```python
from build123d import *

# Parameters (mm, degrees)
F0_R     = 2
F0_R_2   = 12.5
F1_DEPTH = 1


with BuildPart() as f1:
    # F0 (on Top) → F1 (new body)
    with BuildSketch(Plane.XY):
        with BuildLine():
            ThreePointArc((21.15, 16.15), (19.685534, 19.685534), (16.15, 21.15))
            Line((16.15, 21.15), (-16.15, 21.15))
            ThreePointArc((-16.15, 21.15), (-19.685534, 19.685534), (-21.15, 16.15))
            Line((-21.15, 16.15), (-21.15, -16.15))
            ThreePointArc((-21.15, -16.15), (-19.685534, -19.685534), (-16.15, -21.15))
            Line((-16.15, -21.15), (16.15, -21.15))
            ThreePointArc((16.15, -21.15), (19.685534, -19.685534), (21.15, -16.15))
            Line((21.15, -16.15), (21.15, 16.15))
        make_face()
        with Locations((-15.5, -15.5)):
            Circle(F0_R, mode=Mode.SUBTRACT)
        with Locations((15.5, -15.5)):
            Circle(F0_R, mode=Mode.SUBTRACT)
        with Locations((-15.5, 15.5)):
            Circle(F0_R, mode=Mode.SUBTRACT)
        Circle(F0_R_2, mode=Mode.SUBTRACT)
        with Locations((15.5, 15.5)):
            Circle(F0_R, mode=Mode.SUBTRACT)
    extrude(amount=F1_DEPTH)


solid = f1.part
```
Could you check a few things on this model? Use its own coordinates, in mm. Round coordinates to 2 decimals unless told otherwise and drop trailing zeros. Loops run counter-clockwise (first coordinate to the right, second up) from the corner with the lowest first, then second, coordinate; pieces in that order, holes last. Notation, with made-up numbers: M 71,-8.75 L 79,-8.75 A28 cw 79,17.25 Z; hole C 7,-30 d7. An arc over 180 degrees is marked long. Write item = value, one per line.
1. I want a section at D-D, the plane y = 0. Write out the boundary of the cut face in (x, z), and give its area (3 significant figures).
Results below:
outline = M -21.15,0 L -12.5,0 L -12.5,1 L -21.15,1 Z; M 12.5,0 L 21.15,0 L 21.15,1 L 12.5,1 Z
area = 17.3 mm²
2. I want a section at B-B, the plane z = 0.15. Write out the boundary of the cut face in (x, y).
Results below:
outline = M -21.15,-16.15 A5 ccw -16.15,-21.15 L 16.15,-21.15 A5 ccw 21.15,-16.15 L 21.15,16.15 A5 ccw 16.15,21.15 L -16.15,21.15 A5 ccw -21.15,16.15 Z; hole C -15.5,-15.5 d4; hole C -15.5,15.5 d4; hole C 0,0 d25; hole C 15.5,-15.5 d4; hole C 15.5,15.5 d4
3. Thinking about a two-plate mould opening in Y: for faces 1 (the face through (15.24, 17.483, 0.493)), 2 (the face through (9, -9, 0)), 3 (the face through (19.65, -19.72, 0.49)), which applies, +Y half, -Y half, draft (parallel to the pull), parting line (faces both ways), or undercut?
Results below:
face_1 = undercut
face_2 = draft
face_3 = -Y half
4. Will this pin go through, and if not, where does the flat tip stop? P1, Ø2.5, axis at x = 15.5, y = 15.5, coming from the -Z side.
Results below:
P1 = through
5. I want a section at A-A, the plane y = 15.5. Write out the boundary of the cut face in (x, z).
Results below:
outline = M -21.15,0 L -17.5,0 L -17.5,1 L -21.15,1 Z; M -13.5,0 L 13.5,0 L 13.5,1 L -13.5,1 Z; M 17.5,0 L 21.15,0 L 21.15,1 L 17.5,1 Z
6. I need wall thicknesses on probe 1 along Y at (x, z) = (-15.5, 0.5); probe 2 along Y at (x, z) = (14, 0.25). Which ranges of each line are inside material? Lowest first, please.
Results below:
probe_1 = -21.15 to -17.5, -13.5 to 13.5, 17.5 to 21.15
probe_2 = -21.15 to -16.82, -14.18 to 14.18, 16.82 to 21.15
